The model under review builds one solid part; all positions refer to its coordinate system, in mm. Give positions to 0.01 mm unless a question says otherwise; leave off trailing zeros. Order: outer loops, then holes, each group sorted by start corner. A loop starts at its lowest first (then second) coordinate and runs counter-clockwise, first axis right, second up. Notation, with made-up numbers: (18, 60) - (31, 60) arc R30 cw to (31, 98) - close; hole circle Ø10 at (65.25, 30.25). An arc over 180 degrees is marked (long way). Use a Markdown table: item, result. Add a question column.
Autodesk Inventor part; units mm, degrees
ref_plane "Work Plane1" through (7.5, 0, 0) normal (1, 0, 0) x (0, 0, -1)
ref_plane "Work Plane2" through (0, 0, 0) normal (-1, 0, 0) x (0, 0, 1)
ref_plane "YZ Plane" through (0, 0, 0) normal (1, 0, 0) x (0, 1, 0)
sketch "Sketch1" plane through (0, 0, 0) normal (0, 0, 1) x (1, 0, 0)
  line L0 (0, 0) -> (7.5, 0)
  line L1 (7.5, 0) -> (7.5, 3)
  line L2 (7.5, 3) -> (0, 3)
  line L3 (0, 3) -> (0, 0)
  dimension "d0" = 7.5
  dimension "d1" = 3
revolve "Revolution1" add sketch "Sketch1" angle 360 about axis through (0, 0, 0) along (1, 0, 0)
sketch "Sketch2" plane through (0, 0, 0) normal (0, 0, 1) x (1, 0, 0)
  line L0 (7.5, -3) -> (7.5, 3)
  line L1 (7.5, 0) -> (19.8, 0)
  line L2 (20, -0.2) -> (20, -12.5)
  line L3 (0, 0) -> (-12.3, 0)
  line L4 (-12.5, -0.2) -> (-12.5, -12.5)
  arc A0 (-12.3, 0) -> (-12.5, -0.2) centre (-12.3, -0.2) ccw
  arc A1 (20, -0.2) -> (19.8, 0) centre (19.8, -0.2) ccw
  point P0 (20, 0)
  point P1 (-12.5, 0)
  dimension "d3" = 12.5
  dimension "d4" = 12.5
  dimension "d5" = 12.5
  dimension "d6" = 12.5
  dimension "d7" = 0.2
ref_plane "Work Plane1" through (7.5, 0, 0) normal (1, 0, 0) x (0, 0, -1)
ref_plane "Work Plane2" through (0, 0, 0) normal (-1, 0, 0) x (0, 0, 1)
sketch "Sketch3" plane through (7.5, 0, 0) normal (1, 0, 0) x (0, 0, -1)
  circle A0 centre (0, 0) radius 0.25
  dimension "d10" = 0.5
sketch "Sketch4" plane through (0, 0, 0) normal (-1, 0, 0) x (0, 0, 1)
  circle A0 centre (0, 0) radius 0.25
  dimension "d11" = 0.5
sweep "Sweep1" add profiles "Sketch4" path "Sketch2" path curves L3 A0 L4
sweep "Sweep2" add profiles "Sketch3" path "Sketch2" path curves L1 A1 L2
equation "\"BendRadius\" = Thickness"
equation "\"BendReliefWidth\" = Thickness"
equation "\"BendReliefDepth\" = 0.5 * Thickness"
equation "\"CornerReliefSize\" = 4 * Thickness"
equation "\"MinimumRemnant\" = 2 * Thickness"
equation "\"TransitionRadius\" = BendRadius"
equation "\"JacobiRadiusSize\" = BendRadius"
equation "\"GapSize\" = Thickness"
properties part number "KC139"
Q1. We need section A-A (y = -7). Write out the cut boundary in (x, z).
Q2. We need section D-D (y = 1.5). Write out the cut boundary in (x, z), plus the area to 3 significant figures.
Q3. We need section B-B (x = -6.5). Write out the cut boundary in (y, z).
Q4. Clearance check with flat-ended pins moving along their axes: P1, Ø6, axis at x = -8.5, y = -5.5, coming from the -Z side; P2, Ø3, axis at y = 1, z = -0.5, coming from the +X side; P3, Ø1, axis at x = 4, z = 1, coming from the +Y side; P4, Ø3, axis at y = 1.5, z = 1, coming from the -X side. State where each tip first meets the part, or that it passes through.
Q5. We need section C-C (z = 2.4). Write out the cut boundary in (x, y), plus the area to 3 significant figures.
Q6. Wall thickness on probe 1 along X at (y, z) = (-1.75, 1.95); probe 2 along Y at (x, z) = (-10.5, 0.1); probe 3 along Y at (x, z) = (5.5, -0.85): over which ranges is each line inside the solid? List them lowest first.
Here are the results:
| question | item | result |
|---|---|---|
| 1 | outline | circle Ø0.5 at (-12.5, 0); circle Ø0.5 at (20, 0) |
| 2 | outline | (0, -2.6) - (7.5, -2.6) - (7.5, 2.6) - (0, 2.6) - close |
| 2 | area | 39.0 mm2 |
| 3 | outline | circle Ø0.5 at (0, 0) |
| 4 | P1 | through |
| 4 | P2 | x = 20.25 |
| 4 | P3 | y = 2.96 |
| 4 | P4 | x = 0 |
| 5 | outline | (0, -1.8) - (7.5, -1.8) - (7.5, 1.8) - (0, 1.8) - close |
| 5 | area | 27.0 mm2 |
| 6 | probe 1 | 0 to 7.5 |
| 6 | probe 2 | -0.23 to 0.23 |
| 6 | probe 3 | -2.88 to 2.88 |
